from build123d import *

# Parameters (mm, degrees)
SKETCH1_R           = 19
SKETCH1_R_2         = 9
BOSS_EXTRUDE1_DEPTH = 4
CUT_EXTRUDE1_DEPTH  = 4
FILLET1_R           = 0.5


with BuildPart() as part:
    # Sketch1 → Boss-Extrude1 (new body)
    with BuildSketch(Plane.XY):
        Circle(SKETCH1_R)
        Circle(SKETCH1_R_2, mode=Mode.SUBTRACT)
        with BuildLine():
            Line((6.689691504, 12.241024694), (6.226047976, 11.350373764))
            ThreePointArc((6.226047976, 11.350373764), (5.41320923, 10.635157913), (4.330662681, 10.653420143))
            ThreePointArc((4.330662681, 10.653420143), (0, 11.5), (-4.330662681, 10.653420143))
            ThreePointArc((-4.330662681, 10.653420143), (-5.41320923, 10.635157913), (-6.226047976, 11.350373764))
            Line((-6.226047976, 11.350373764), (-6.689691504, 12.241024694))
            ThreePointArc((-6.689691504, 12.241024694), (-6.768746058, 13.446590252), (-5.933372603, 14.319395572))
            ThreePointArc((-5.933372603, 14.319395572), (0, 15.5), (5.933372603, 14.319395572))
            ThreePointArc((5.933372603, 14.319395572), (6.768746058, 13.446590252), (6.689691504, 12.241024694))
        make_face(mode=Mode.SUBTRACT)
        with BuildLine():
            Line((12.241024694, 6.689691504), (11.350373764, 6.226047976))
            ThreePointArc((11.350373764, 6.226047976), (10.635157913, 5.41320923), (10.653420143, 4.330662681))
            ThreePointArc((10.653420143, 4.330662681), (11.5, 0), (10.653420143, -4.330662681))
            ThreePointArc((10.653420143, -4.330662681), (10.635157913, -5.41320923), (11.350373764, -6.226047976))
            Line((11.350373764, -6.226047976), (12.241024694, -6.689691504))
            ThreePointArc((12.241024694, -6.689691504), (13.446590252, -6.768746058), (14.319395572, -5.933372603))
            ThreePointArc((14.319395572, -5.933372603), (15.5, 0), (14.319395572, 5.933372603))
            ThreePointArc((14.319395572, 5.933372603), (13.446590252, 6.768746058), (12.241024694, 6.689691504))
        make_face(mode=Mode.SUBTRACT)
        with BuildLine():
            Line((6.689691504, -12.241024694), (6.226047976, -11.350373764))
            ThreePointArc((6.226047976, -11.350373764), (5.41320923, -10.635157913), (4.330662681, -10.653420143))
            ThreePointArc((4.330662681, -10.653420143), (0, -11.5), (-4.330662681, -10.653420143))
            ThreePointArc((-4.330662681, -10.653420143), (-5.41320923, -10.635157913), (-6.226047976, -11.350373764))
            Line((-6.226047976, -11.350373764), (-6.689691504, -12.241024694))
            ThreePointArc((-6.689691504, -12.241024694), (-6.768746058, -13.446590252), (-5.933372603, -14.319395572))
            ThreePointArc((-5.933372603, -14.319395572), (0, -15.5), (5.933372603, -14.319395572))
            ThreePointArc((5.933372603, -14.319395572), (6.768746058, -13.446590252), (6.689691504, -12.241024694))
        make_face(mode=Mode.SUBTRACT)
        with BuildLine():
            Line((-12.241024694, -6.689691504), (-11.350373764, -6.226047976))
            ThreePointArc((-11.350373764, -6.226047976), (-10.635157913, -5.41320923), (-10.653420143, -4.330662681))
            ThreePointArc((-10.653420143, -4.330662681), (-11.5, 0), (-10.653420143, 4.330662681))
            ThreePointArc((-10.653420143, 4.330662681), (-10.635157913, 5.41320923), (-11.350373764, 6.226047976))
            Line((-11.350373764, 6.226047976), (-12.241024694, 6.689691504))
            ThreePointArc((-12.241024694, 6.689691504), (-13.446590252, 6.768746058), (-14.319395572, 5.933372603))
            ThreePointArc((-14.319395572, 5.933372603), (-15.5, 0), (-14.319395572, -5.933372603))
            ThreePointArc((-14.319395572, -5.933372603), (-13.446590252, -6.768746058), (-12.241024694, -6.689691504))
        make_face(mode=Mode.SUBTRACT)
    extrude(amount=BOSS_EXTRUDE1_DEPTH)

    # Sketch2 → Cut-Extrude1 (cut)
    with BuildSketch(Plane(origin=(0, 0, 0), x_dir=(-1, 0, 0), z_dir=(0, 0, -1))):
        Polygon((10.65368142, -8.367490994), (8.367490994, -10.65368142), (9.204294768, -13.776675621), (12.327288968, -14.613479395), (14.613479395, -12.327288968), (13.776675621, -9.204294768), align=None)
        Polygon((13.776675621, 9.204294768), (14.613479395, 12.327288968), (12.327288968, 14.613479395), (9.204294768, 13.776675621), (8.367490994, 10.65368142), (10.65368142, 8.367490994), align=None)
        Polygon((-8.367490994, -10.65368142), (-10.65368142, -8.367490994), (-13.776675621, -9.204294768), (-14.613479395, -12.327288968), (-12.327288968, -14.613479395), (-9.204294768, -13.776675621), align=None)
        Polygon((-10.65368142, 8.367490994), (-8.367490994, 10.65368142), (-9.204294768, 13.776675621), (-12.327288968, 14.613479395), (-14.613479395, 12.327288968), (-13.776675621, 9.204294768), align=None)
    extrude(amount=-CUT_EXTRUDE1_DEPTH, mode=Mode.SUBTRACT)

    # Fillet1
    fillet1_edges = [part.edges().sort_by_distance(p)[0] for p in [
        (-9, 0, 0),
        (-9, 0, 4),
    ]]
    fillet(fillet1_edges, radius=FILLET1_R)


solid = part.part
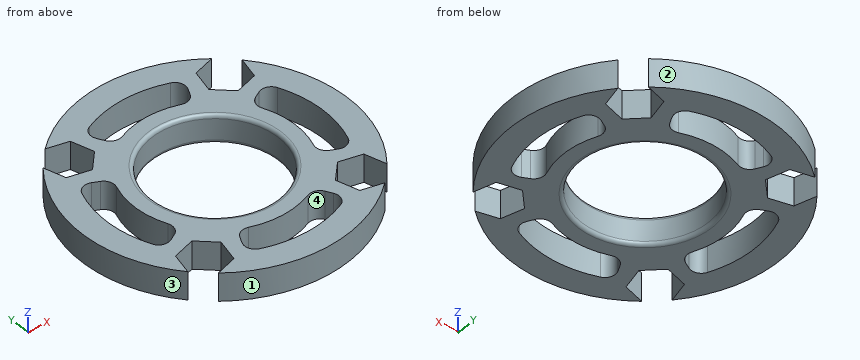
Work out the finished part from the listing and answer in its coordinate system (mm). Face numbers are marked on the shaded views. Give positions to 0.01 mm unless a question says otherwise; leave off trailing zeros. Loops run counter-clockwise (first coordinate to the right, second up) from the corner with the lowest first, then second, coordinate; pieces in that order, holes last. Notation, with made-up numbers: (5, -14.5) - (23, -14.5) arc R28 ccw to (23, 18.5) - close; hole circle Ø9 at (-14.75, 0.25). An arc over 180 degrees is marked (long way). Answer in a Markdown table with one row per item. Add a question column.
Q1. The part is cut by section D-D (z = 3.05). State how many separate pieces and enclosed holes the cut face has, and give its area (3 significant figures).
Q2. The part is cut by section A-A (y = 0). Determine the outline of the cut face in (x, z).
Q3. Consider line 1 along Y through (x, z) = (0, 1.6); line 2 along Y through (x, z) = (1, 0.9); line 3 along X through (y, z) = (2.5, 2.05). Determine where each line is inside the solid, lowest interval first.
Q4. Each of these flat-tipped pins is pushed along its axis until it touches: P1, Ø11, axis at x = 0, y = 0, coming from the -Z side; P2, Ø1, axis at x = -12, z = 2.5, coming from the -Y side. Where does it stop, or does it pass through?
Q5. The part is cut by section C-C (y = -10). Determine the outline of the cut face in (x, z), and give its area (3 significant figures).
Q6. Determine the mould class of the marked faces 1, 2, 3 and 4 for opening direction Y: released by +Y, released by -Y, zero draft, split by the parting line, or undercut.
Solution:
| question | item | result |
|---|---|---|
| 1 | separate pieces | 1 |
| 1 | enclosed holes | 5 |
| 1 | area | 563 mm² |
| 2 | outline | (-19, 0) - (-15.5, 0) - (-15.5, 4) - (-19, 4) - close; (-11.5, 0) - (-9.5, 0) arc R0.5 ccw to (-9, 0.5) - (-9, 3.5) arc R0.5 ccw to (-9.5, 4) - (-11.5, 4) - close; (9, 0.5) arc R0.5 ccw to (9.5, 0) - (11.5, 0) - (11.5, 4) - (9.5, 4) arc R0.5 ccw to (9, 3.5) - close; (15.5, 0) - (19, 0) - (19, 4) - (15.5, 4) - close |
| 3 | line 1 | y = -19 to -15.5, -11.5 to -9, 9 to 11.5, 15.5 to 19 |
| 3 | line 2 | y = -18.97 to -15.47, -11.46 to -8.94, 8.94 to 11.46, 15.47 to 18.97 |
| 3 | line 3 | x = -18.83 to -15.3, -11.22 to -8.65, 8.65 to 11.22, 15.3 to 18.83 |
| 4 | P1 | passes through |
| 4 | P2 | stops at y = -15.12 |
| 5 | outline | (-16.16, 0) - (-13.99, 0) - (-13.99, 4) - (-16.16, 4) - close; (-9.02, 0) - (9.02, 0) - (9.02, 4) - (-9.02, 4) - close; (13.99, 0) - (16.16, 0) - (16.16, 4) - (13.99, 4) - close |
| 5 | area | 89.5 mm² |
| 6 | face 1 | released by -Y |
| 6 | face 2 | released by +Y |
| 6 | face 3 | split by the parting line |
| 6 | face 4 | undercut |
